Read the model definition and answer for the solid it produces. Units are mm, in the model's axes. A direction names the side the tool comes from. Give positions to 0.01 mm unless a question says otherwise; leave off trailing zeros. Order: outer loops, then holes, each group sorted by start corner. A loop starts at its lowest first (then second) coordinate and runs counter-clockwise, first axis right, second up. Notation, with made-up numbers: (40.25, -33) - (74.25, -33) arc R16 cw to (74.25, -20) - close; hole circle Ø7 at (-18.5, 16). An arc over 180 degrees is marked (long way). Write item = value, one per line.
```python
from build123d import *

# Parameters (mm, degrees)
F0_R     = 2.499999
F0_W     = 12
F0_H     = 37.150002
F1_DEPTH = 15
F2_W     = 10
F2_H     = 15
F3_DEPTH = 8
F4_R     = 2


with BuildPart() as f1:
    # F0 (on Top) → F1 (new body)
    with BuildSketch(Plane.XY):
        with BuildLine():
            Line((46.450001, 45.150002), (8.95, 45.150002))
            Line((8.95, 45.150002), (8.95, 30.300001))
            Line((8.95, 30.300001), (10.099999, 29.150002))
            Line((10.099999, 29.150002), (10.099999, 7.5))
            ThreePointArc((10.099999, 7.5), (12.296699, 2.196699), (17.599999, 0))
            Line((17.599999, 0), (37.799999, 0))
            ThreePointArc((37.799999, 0), (43.1033, 2.196699), (45.299999, 7.5))
            Line((45.299999, 7.5), (45.299999, 29.150002))
            Line((45.299999, 29.150002), (46.450001, 30.300001))
            Line((46.450001, 30.300001), (46.450001, 45.150002))
        make_face()
        with Locations((16.199999, 7.749999)):
            Circle(F0_R, mode=Mode.SUBTRACT)
        with Locations((39.199598, 7.749999)):
            Circle(F0_R, mode=Mode.SUBTRACT)
        with Locations((16.199999, 30.749999)):
            Circle(F0_R, mode=Mode.SUBTRACT)
        with Locations((27.700001, 22.575001)):
            Rectangle(F0_W, F0_H, mode=Mode.SUBTRACT)
        with Locations((39.199598, 30.749999)):
            Circle(F0_R, mode=Mode.SUBTRACT)
    extrude(amount=F1_DEPTH)

    # F2 (on face) → F3 (join)
    with BuildSketch(Plane(origin=(10.099999, 0, 0), x_dir=(0, -1, 0), z_dir=(-1, 0, 0))):
        with Locations((-14.181, 7.5)):
            Rectangle(F2_W, F2_H)
    extrude(amount=F3_DEPTH)

    # F4
    f4_edges = [f1.edges().sort_by_distance(p)[0] for p in [
        (2.099999, 19.181, 7.5),
        (2.099999, 9.181, 7.5),
    ]]
    fillet(f4_edges, radius=F4_R)


solid = f1.part
```
1. Determine the mould class of faces 5 (the face through (33.7, 22, 7)), 6 (the face through (2.7, 18.61, 7.6)), 7 (the face through (46.45, 38, 7)), 8 (the face through (28, 0, 7)) for opening direction Y: +Y half, -Y half, draft (parallel to the pull), parting line (faces both ways), or undercut.
Recorded:
face_5 = undercut
face_6 = +Y half
face_7 = draft
face_8 = -Y half
2. Straight lines are drawn through the part: L1, parallel to X at y = 41, z = 4; L2, parallel to Y at x = 28, z = 14.5; L3, parallel to X at y = 27, z = 3.5. For each, find the intervals that lie inside material, in ascending order. Write a range as [from, to].
Recorded:
L1 = [8.95, 21.7], [33.7, 46.45]
L2 = [0, 4], [41.15, 45.15]
L3 = [10.1, 21.7], [33.7, 45.3]
3. Section B-B (x = 15.5) is taken. Determine the outline of the cut face in (y, z), and give its area (3 significant figures).
Recorded:
outline = (0.3, 0) - (5.35, 0) - (5.35, 15) - (0.3, 15) - close; (10.15, 0) - (28.35, 0) - (28.35, 15) - (10.15, 15) - close; (33.15, 0) - (45.15, 0) - (45.15, 15) - (33.15, 15) - close
area = 529 mm^2
4. Section A-A (y = 21) is taken. Determine the outline of the cut face in (x, z), and give its area (3 significant figures).
Recorded:
outline = (10.1, 0) - (21.7, 0) - (21.7, 15) - (10.1, 15) - close; (33.7, 0) - (45.3, 0) - (45.3, 15) - (33.7, 15) - close
area = 348 mm^2
5. Section C-C (z = 10.25) is taken. Determine the outline of the cut face in (x, y), and give its area (3 significant figures).
Recorded:
outline = (2.1, 11.18) arc R2 ccw to (4.1, 9.18) - (10.1, 9.18) - (10.1, 7.5) arc R7.5 ccw to (17.6, 0) - (37.8, 0) arc R7.5 ccw to (45.3, 7.5) - (45.3, 29.15) - (46.45, 30.3) - (46.45, 45.15) - (8.95, 45.15) - (8.95, 30.3) - (10.1, 29.15) - (10.1, 19.18) - (4.1, 19.18) arc R2 ccw to (2.1, 17.18) - close; hole circle Ø5 at (16.2, 7.75); hole circle Ø5 at (16.2, 30.75); hole (21.7, 4) - (33.7, 4) - (33.7, 41.15) - (21.7, 41.15) - close; hole circle Ø5 at (39.2, 7.75); hole circle Ø5 at (39.2, 30.75)
area = 1,150 mm^2
6. Section D-D (x = 31) is taken. Determine the outline of the cut face in (y, z), and give its area (3 significant figures).
Recorded:
outline = (0, 0) - (4, 0) - (4, 15) - (0, 15) - close; (41.15, 0) - (45.15, 0) - (45.15, 15) - (41.15, 15) - close
area = 120 mm^2
7. For faces 1 (the face through (2.1, 14, 8)), 2 (the face through (7, 9.181, 7)), 3 (the face through (9.52, 29.73, 7.4)), 4 (the face through (28, 4, 7)), determine the directions among +Z, -Z, +X, -X, +Y, -Y from which every point of the face is accessible in a straight line to the end or side of a thin tool.
Recorded:
face_1 = +Z, -Z, -X, +Y, -Y
face_2 = +Z, -Z, -X, -Y
face_3 = +Z, -Z, -X
face_4 = +Z, -Z
8. Flat-ended cylindrical pins translate along their axes: pin 1 (6.5 mm diameter, centred on x = 7, z = 6, fed in from +Y); pin 2 (3 mm diameter, centred on y = 22.5, z = 10.5, fed in from -X); pin 3 (4.5 mm diameter, centred on y = 29, z = 4, fed in from -X); pin 4 (3 mm diameter, centred on x = 8, z = 4, fed in from -Y). Find the tip coordinate at first contact, or state that the pin passes through.
Recorded:
pin_1 = 45.15
pin_2 = 10.1
pin_3 = 8.95
pin_4 = 9.18
